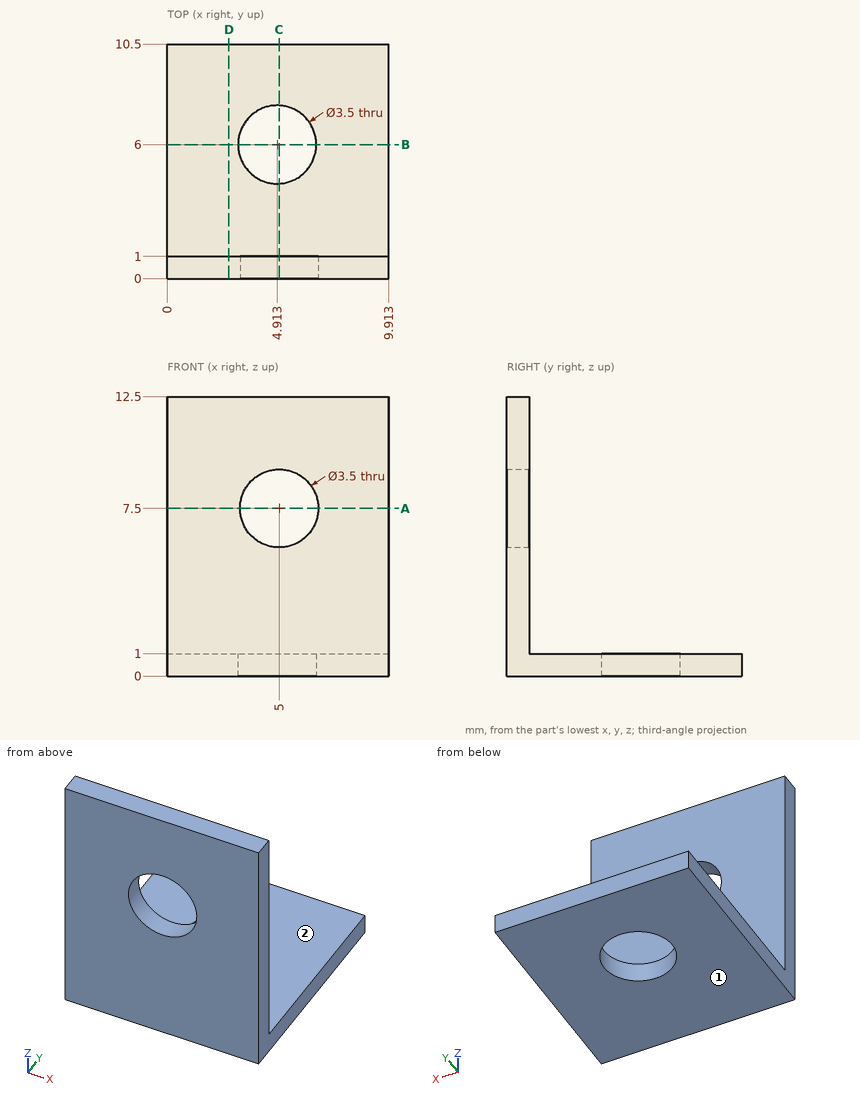
Check sheet for the drawn part. Datum: minimum x, y, z corner. Units: mm. A direction names the side the tool comes from. Round coordinates to 2 decimals unless told otherwise and drop trailing zeros. Order: outer loops, then holes, each group sorted by start corner. A loop starts at its lowest first (then second) coordinate and runs counter-clockwise, first axis right, second up. Notation, with made-up numbers: M -11,73.5 L 19,73.5 A17 cw 19,100.5 Z; hole C 24.5,40.25 d10. An arc over 180 degrees is marked long. Write each question's results on one line, items separated by ' | '. Start each with the question number.
1. Set-up check for the marked faces 1 and 2: record each of +Z, -Z, +X, -X, +Y, -Y from which the full face is reachable in a straight line by a thin tool's end or side.
2. Go/stop test with flat-tipped pins: P1, Ø5, axis at x = 5.5, y = 7.5, coming from the +Z side; P2, Ø5, axis at x = 4, z = 7.5, coming from the +Y side; P3, Ø1.5, axis at x = 3, z = 6, coming from the -Y side. Record where each tip stops, or that it passes through.
3. Cross-section at A-A on z = 7.5. Record the boundary of the cut face in (x, y).
4. Cross-section at D-D on x = 2.75. Record the boundary of the cut face in (y, z), plus the area to 3 significant figures.
5. Material ranges on L1, parallel to X at y = 0.65, z = 7.5; L2, parallel to Z at x = 6.5, y = 3, recorded low to high. Write a range as from..to.
6. Cross-section at B-B on y = 6. Record the boundary of the cut face in (x, z).
7. Cross-section at C-C on x = 5. Record the boundary of the cut face in (y, z).
Resolved:
1) face 1: -Z, +X, -X, +Y, -Y | face 2: +Z, +X, -X, +Y
2) P1: z = 1 | P2: y = 1 | P3: y = 0
3) outline: M 0,0 L 3.25,0 L 3.25,1 L 0,1 Z; M 6.75,0 L 9.91,0 L 9.91,1 L 6.75,1 Z
4) outline: M 0,0 L 10.5,0 L 10.5,1 L 1,1 L 1,12.5 L 0,12.5 Z | area: 22.0 mm2
5) L1: 0..3.25, 6.75..9.91 | L2: 0..1
6) outline: M 0,0 L 3.16,0 L 3.16,1 L 0,1 Z; M 6.66,0 L 9.91,0 L 9.91,1 L 6.66,1 Z
7) outline: M 0,0 L 4.25,0 L 4.25,1 L 1,1 L 1,5.75 L 0,5.75 Z; M 0,9.25 L 1,9.25 L 1,12.5 L 0,12.5 Z; M 7.75,0 L 10.5,0 L 10.5,1 L 7.75,1 Z
